from build123d import *

# Parameters (mm, degrees)
F1_DEPTH = 19.05
F2_DEPTH = 3.175
F3_R     = 6.35
F4_R     = 2.53999
F5_R     = 2.54


# Not quite as in the source:
# - a fillet or chamfer is up to 0.001 mm smaller than in the source, because OpenCascade refuses the exact size


with BuildPart() as f1:
    # F0 (on Front) → F1 (new body)
    with BuildSketch(Plane.XZ):
        Polygon((-33.02, 0), (0, 0), (5.08, 0), (5.08, 5.08), (5.08, 58.42), (38.1, 58.42), (38.1, 63.5), (5.08, 63.5), (0, 63.5), (0, 58.42), (0, 5.08), (-33.02, 5.08), align=None)
    extrude(amount=F1_DEPTH)

    # F0 (on Front) → F2 (join)
    with BuildSketch(Plane.XZ):
        with BuildLine():
            Line((5.08, 0), (0, 0))
            Line((0, 0), (-33.02, 0))
            ThreePointArc((-33.02, 0), (-31.1601280605, -4.4901280605), (-26.67, -6.35))
            Line((-26.67, -6.35), (7.3484978099, -6.35))
            ThreePointArc((7.3484978099, -6.35), (10.7819271621, -5.3417284546), (13.1250166344, -2.6371064199))
            Line((13.1250166344, -2.6371064199), (37.5265188245, 50.8138031394))
            ThreePointArc((37.5265188245, 50.8138031394), (37.9549735912, 52.1015383235), (38.1, 53.4509095593))
            Line((38.1, 53.4509095593), (38.1, 58.42))
            Line((38.1, 58.42), (5.08, 58.42))
            Line((5.08, 58.42), (5.08, 5.08))
            Line((5.08, 5.08), (5.08, 0))
        make_face()
    extrude(amount=F2_DEPTH)

    # F3
    f3_edges = [f1.edges().sort_by_distance(p)[0] for p in [
        (0, -9.525, 63.5),
        (5.08, -11.1125, 0),
    ]]
    fillet(f3_edges, radius=F3_R)

    # F4 (radius 2.54 in the source; OpenCascade refuses exactly that, so slightly less here)
    f4_edges = [f1.edges().sort_by_distance(p)[0] for p in [
        (-33.02, -11.1125, 0),
        (-33.02, -1.5875, 0),
        (-33.02, -9.525, 5.08),
        (38.1, -11.1125, 58.42),
        (38.1, -9.525, 63.5),
    ]]
    fillet(f4_edges, radius=F4_R)

    # F5
    f5_edges = [f1.edges().sort_by_distance(p)[0] for p in [
        (5.08, -11.1125, 58.42),
        (0, -9.525, 5.08),
    ]]
    fillet(f5_edges, radius=F5_R)


solid = f1.part
Could you check a few things on this model? Use its own coordinates, in mm. A direction names the side the tool comes from. Coordinates: 2 decimals unless noted, no trailing zeros. Write each loop counter-clockwise with the first axis right and the second up, starting at its lowest first coordinate (ties: lowest second). Pieces come first, ordered by that corner, then holes. Notation, with made-up numbers: (27.25, 52) - (67.25, 52) arc R17 ccw to (67.25, 59) - close; hole circle Ø5 at (-4, 26.25). An arc over 180 degrees is marked (long way). Put each result on its own line as item: value. Start each with the question number.
Q1. Which directions (+Z, -Z, +X, -X, +Y, -Y) give clear straight access to the entire face, cutting with the end or side of a thin tool? Please do faces 1 (the flat face through (-16, -11, 0)), 2 (the cylindrical face through (-32.256, -11.224, 0.724)), 3 (the flat face through (-16, -9, 5.08)), 4 (the cylindrical face through (37.336, -11.224, 59.144)).
Q2. Please list where these lines run through material, in increasing order: L1, parallel to Y at x = 18.5, z = 48 (3 decimals); L2, parallel to Z at x = 14.5, y = -18; L3, parallel to X at y = -10, z = 12.
Q3. I want a section at C-C on x = 15. Write out the boundary of the cut face in (y, z) (3 decimals), plus the area to 3 significant figures.
Q4. I'm going to push flat-ended pins straight in: P1, Ø2, axis at y = -15.5, z = 4, coming from the -X side; P2, Ø1.5, axis at x = -10, y = -6, coming from the +Z side; P3, Ø1, axis at y = -16, z = 38.5, coming from the -X side. Where does each tip first touch, or does it pass through?
Q5. I want a section at B-B on z = 55. Write out the boundary of the cut face in (x, y) (3 decimals), plus the area to 3 significant figures.
Checks:
1. face 1: -Z, +X, -X, -Y
1. face 2: -Z, -X, -Y
1. face 3: +Z, -X, +Y, -Y
1. face 4: -Z, +X, -Y
2. L1: -3.175 to 0
2. L2: 58.42 to 63.5
2. L3: 0 to 5.08
3. outline: (-19.05, 58.42) - (-3.175, 58.42) - (-3.175, 1.47) - (0, 1.47) - (0, 63.5) - (-19.05, 63.5) - close
3. area: 278 mm²
4. P1: x = -32.98
4. P2: z = 5.08
4. P3: x = 0
5. outline: (0, -19.05) - (5.08, -19.05) - (5.08, -3.175) - (38.1, -3.175) - (38.1, 0) - (0, 0) - close
5. area: 202 mm²
